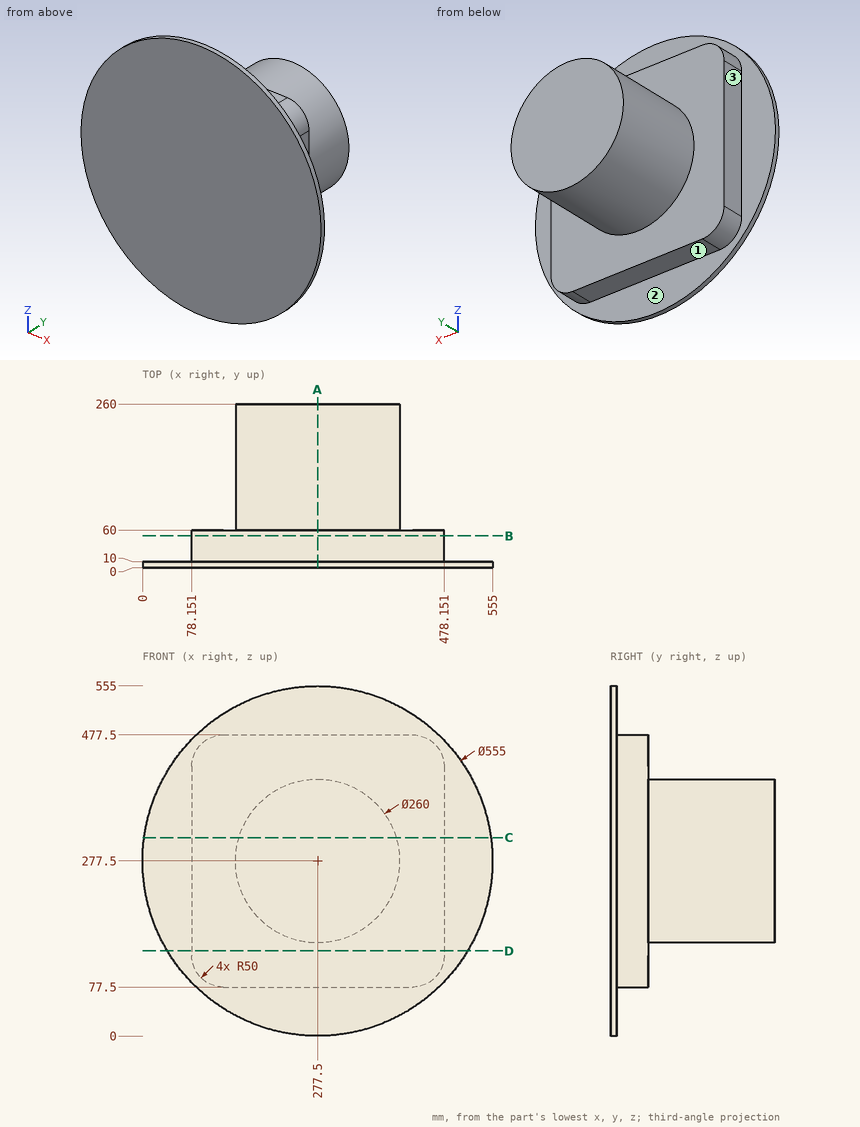
Could you check a few things on this drawing? It's one solid part, dimensions in mm from its lowest x, y, z. A direction names the side the tool comes from. Coordinates: 2 decimals unless noted, no trailing zeros. Write each loop counter-clockwise with the first axis right and the second up, starting at its lowest first coordinate (ties: lowest second). Pieces come first, ordered by that corner, then holes. Notation, with made-up numbers: (46.5, 60) - (60.5, 60) arc R24 cw to (60.5, 87) - close; hole circle Ø1 at (4.5, 77.25). An arc over 180 degrees is marked (long way). Write item = value, one per line.
1) For the marked faces 1, 2 and 3, which set-ups out of +Z, -Z, +X, -X, +Y, -Y let a thin tool reach every point of the face, with its end or its side?
Result set:
face_1 = -Z, +X, -X, +Y
face_2 = +Y
face_3 = +Z, -Z, -X, +Y
2) Suppose I cut it at C-C on z = 314.5. Please give me the cut outline in (x, y).
Result set:
outline = (2.48, 0) - (552.52, 0) - (552.52, 10) - (478.15, 10) - (478.15, 60) - (402.12, 60) - (402.12, 260) - (152.88, 260) - (152.88, 60) - (78.15, 60) - (78.15, 10) - (2.48, 10) - close
3) Suppose I cut it at A-A on x = 277.5. Please give me the cut outline in (y, z), plus the area to 4 significant figures.
Result set:
outline = (0, 0) - (10, 0) - (10, 77.5) - (60, 77.5) - (60, 147.5) - (260, 147.5) - (260, 407.5) - (60, 407.5) - (60, 477.5) - (10, 477.5) - (10, 555) - (0, 555) - close
area = 77,550 mm2
4) Suppose I cut it at B-B on y = 51. Please give me the cut outline in (x, z).
Result set:
outline = (78.15, 127.5) arc R50 ccw to (128.15, 77.5) - (428.15, 77.5) arc R50 ccw to (478.15, 127.5) - (478.15, 427.5) arc R50 ccw to (428.15, 477.5) - (128.15, 477.5) arc R50 ccw to (78.15, 427.5) - close
5) Please list where these lines run through material, in increasing order: line 1 (Y direction, x = 368, z = 87); line 2 (X direction, y = 55, z = 268); line 3 (Y direction, x = 519, z = 182). Write a range as [from, to].
Result set:
line_1 = [0, 60]
line_2 = [78.15, 478.15]
line_3 = [0, 10]
6) Suppose I cut it at D-D on z = 135. Please give me the cut outline in (x, y).
Result set:
outline = (39.38, 0) - (515.62, 0) - (515.62, 10) - (478.15, 10) - (478.15, 60) - (78.15, 60) - (78.15, 10) - (39.38, 10) - close
7) Will these pins go through, and if not, where does the flat tip stop? pin 1 Ø4 at (x, y) = (182, 28) entering from -Z; pin 2 Ø10 at (y, z) = (42, 149) entering from -X; pin 3 Ø4 at (y, z) = (136, 296) entering from +X.
Result set:
pin_1 = 77.5
pin_2 = 78.15
pin_3 = 406.45
